```python
from build123d import *

# Parameters (mm, degrees)
SKETCH2_W          = 2.5
SKETCH2_H          = 3.5
CUT_EXTRUDE1_DEPTH = 3.5
FILLET1_R          = 0.5
CUT_EXTRUDE2_DEPTH = 0.5


with BuildPart() as part:
    # Sketch1 → Revolve1 (revolve)
    with BuildSketch(Plane.XY, mode=Mode.PRIVATE) as revolve1_sk:
        Polygon((0, 7.25), (5, 7.25), (5, 1.25), (8, 1.25), (8, 0), (0, 0), align=None)
    revolve(revolve1_sk.sketch.rotate(Axis((0, 7.25, 0), (0, -1, 0)), 180), axis=Axis((0, 7.25, 0), (0, -1, 0)))

    # Sketch2 → Cut-Extrude1 (cut)
    with BuildSketch(Plane.XZ):
        Rectangle(SKETCH2_W, SKETCH2_H)
    extrude(amount=-CUT_EXTRUDE1_DEPTH, mode=Mode.SUBTRACT)

    # Fillet1
    fillet1_edges = [part.edges().sort_by_distance(p)[0] for p in [
        (5, 7.25, 0),
    ]]
    fillet(fillet1_edges, radius=FILLET1_R)

    # Sketch3 → Cut-Extrude2 (cut)
    with BuildSketch(Plane(origin=(0, 7.25, 0), x_dir=(1, 0, 0), z_dir=(0, 1, 0))):
        Polygon((-0.972355769, 3), (0.692307692, 3), (0.692307692, -3), (-0.384615385, -3), (-0.384615385, 2), (-1.615384615, 2), align=None)
    extrude(amount=-CUT_EXTRUDE2_DEPTH, mode=Mode.SUBTRACT)


solid = part.part
```
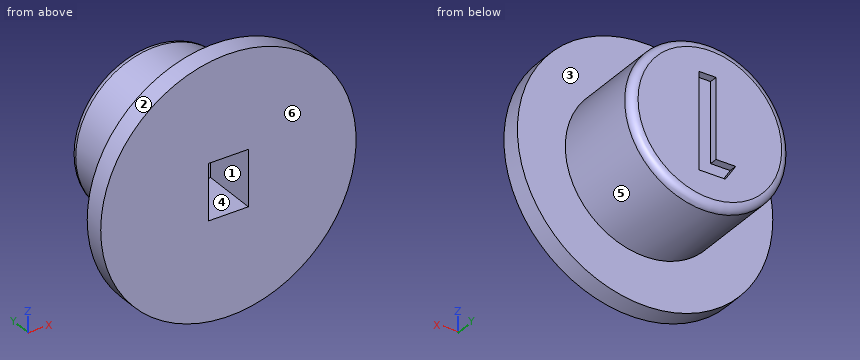
Check sheet for the modelled part. Datum: model origin and axes. Units: mm. Face numbers are marked on the shaded views. A direction names the side the tool comes from. Coordinates: 2 decimals unless noted, no trailing zeros. Write each loop counter-clockwise with the first axis right and the second up, starting at its lowest first coordinate (ties: lowest second). Pieces come first, ordered by that corner, then holes. Notation, with made-up numbers: M -24.5,-19 L 30.5,-19 A20 cw 30.5,-8 Z; hole C 19.25,26.5 d1. An arc over 180 degrees is marked long. Write item = value, one per line. Start each with the question number.
1. Sectioned sample at C-C (y = 1.75). Record the cut outline in (x, z).
2. Tool access check on the marked faces 1, 2 and 3. Record the directions out of +Z, -Z, +X, -X, +Y, -Y that give a thin tool (end or side, any length) a straight path to the whole face; none if there is none.
3. Go/stop test with flat-tipped pins: pin 1 (1 mm diameter, centred on y = 1.5, z = 1, fed in from +X); pin 2 (0.6 mm diameter, centred on y = 7, z = 1, fed in from -X); pin 3 (1 mm diameter, centred on y = 1.5, z = -4.5, fed in from -X). Record where each tip stops, or that it passes through.
4. Thickness scan on probe 1 along Y at (x, z) = (-5.5, 2.5); probe 2 along X at (y, z) = (0.5, -1.25); probe 3 along X at (y, z) = (6, -4). Record the ranges inside material, lowest first.
5. Sectioned sample at A-A (x = 0). Record the cut outline in (y, z).
6. Mould release check, pull along X, two halves, no side actions. Record for the marked faces 4, 5 and 6: pulls with the +X half, pulls with the -X half, needs draft (parallel to the pull), parting line crosses it, or undercut.
7. Sectioned sample at D-D (z = 7.25). Record the cut outline in (x, y).
8. Sectioned sample at B-B (z = 0). Record the cut outline in (x, y).
The answers:
q1.outline = C 0,0 d10; hole M -1.25,-1.75 L 1.25,-1.75 L 1.25,1.75 L -1.25,1.75 Z
q2.face_1 = -Y
q2.face_2 = +Y, -Y
q2.face_3 = +Y
q3.pin_1 = 7.98
q3.pin_2 = -4.94
q3.pin_3 = -6.89
q4.probe_1 = 0 to 1.25
q4.probe_2 = -7.9 to -1.25, 1.25 to 7.9
q4.probe_3 = -3 to 3
q5.outline = M 0,-8 L 1.25,-8 L 1.25,-5 L 6.75,-5 A0.5 ccw 7.25,-4.5 L 7.25,-3 L 6.75,-3 L 6.75,3 L 7.25,3 L 7.25,4.5 A0.5 ccw 6.75,5 L 1.25,5 L 1.25,8 L 0,8 L 0,1.75 L 3.5,1.75 L 3.5,-1.75 L 0,-1.75 Z
q6.face_4 = undercut
q6.face_5 = parting line crosses it
q6.face_6 = needs draft
q7.outline = M -3.38,0 L 3.38,0 L 3.38,1.25 L -3.38,1.25 Z
q8.outline = M -8,0 L -1.25,0 L -1.25,3.5 L 1.25,3.5 L 1.25,0 L 8,0 L 8,1.25 L 5,1.25 L 5,6.75 A0.5 ccw 4.5,7.25 L 0.69,7.25 L 0.69,6.75 L -0.38,6.75 L -0.38,7.25 L -4.5,7.25 A0.5 ccw -5,6.75 L -5,1.25 L -8,1.25 Z
